For this review, take the finished solid that the model builds, in its own axes (mm). A direction names the side the tool comes from. Give positions to 0.01 mm unless a question says otherwise; leave off trailing zeros. Loops run counter-clockwise (first coordinate to the right, second up) from the corner with the lowest first, then second, coordinate; pieces in that order, holes last.
```python
from build123d import *

# Parameters (mm, degrees)
F0_W     = 50.8
F0_H     = 50.8
F1_DEPTH = 50.8
F3_DEPTH = 50.8


with BuildPart() as f1:
    # F0 (on Front) → F1 (new body)
    with BuildSketch(Plane.XZ):
        with Locations((-25.4, 25.4)):
            Rectangle(F0_W, F0_H)
    extrude(amount=F1_DEPTH)

    # F2 (on face) → F3 (intersect)
    with BuildSketch(Plane.XZ.offset(50.8)):
        Polygon((-38.1, 50.8), (-50.8, 50.8), (-50.8, 14.321598), (0, 14.321598), (0, 50.8), (-12.7, 50.8), (-12.7, 25.4), (-38.1, 25.4), align=None)
    extrude(amount=-F3_DEPTH, mode=Mode.INTERSECT)


solid = f1.part
```
Item 1: Tool access review of faces 5 (the flat face through (-26, -26, 14.322)), 6 (the flat face through (-25, -26, 25.4)): name each direction out of +Z, -Z, +X, -X, +Y, -Y from which nothing blocks a thin tool from reaching the whole face with its end or side.
Answer:
face 5: -Z, +X, -X, +Y, -Y
face 6: +Z, +Y, -Y
Item 2: Clearance check with a flat-ended pin moving along its axis: pin 1 Ø5 at (x, y) = (-36.5, -17) entering from +Z. State where the tip first meets the part, or that it passes through.
Answer:
pin 1: stops at z = 50.8
Item 3: For L1, parallel to X at y = -11.5, z = 38; L2, parallel to Z at x = -16, y = -34, list the stretches that pass through material, from the lowest coordinate up.
Answer:
L1: x = -50.8 to -38.1, -12.7 to 0
L2: z = 14.32 to 25.4
Item 4: Take a section at C-C on x = -19. Give the boundary of the cut face in (y, z).
Answer:
outline: (-50.8, 14.32) - (0, 14.32) - (0, 25.4) - (-50.8, 25.4) - close
Item 5: Take a section at A-A on y = -33. Give the boundary of the cut face in (x, z).
Answer:
outline: (-50.8, 14.32) - (0, 14.32) - (0, 50.8) - (-12.7, 50.8) - (-12.7, 25.4) - (-38.1, 25.4) - (-38.1, 50.8) - (-50.8, 50.8) - close
Item 6: Take a section at B-B on z = 46. Give the boundary of the cut face in (x, y), and give its area (3 significant figures).
Answer:
outline: (-50.8, -50.8) - (-38.1, -50.8) - (-38.1, 0) - (-50.8, 0) - close; (-12.7, -50.8) - (0, -50.8) - (0, 0) - (-12.7, 0) - close
area: 1,290 mm2
Item 7: The part is to be moulded in two halves that separate along X. For faces 1 (the flat face through (0, -25, 32)), 2 (the flat face through (-50.8, -25, 32)), 3 (the flat face through (-26, -50.8, 25)), 4 (the flat face through (-12.7, -26, 38)), say which applies: released by +X, released by -X, zero draft, split by the parting line, or undercut.
Answer:
face 1: released by +X
face 2: released by -X
face 3: zero draft
face 4: undercut
